```python
from build123d import *

# Parameters (mm, degrees)
F1_DEPTH = 6
F3_D     = 6
F4_W     = 63.5
F4_H     = 140
F5_DEPTH = 25


with BuildPart() as f1:
    # F0 (on Front) → F1 (new body)
    with BuildSketch(Plane.XZ):
        with BuildLine():
            Line((34.0407285993, 33.1888695754), (-82.9592714007, 33.1888695754))
            ThreePointArc((-82.9592714007, 33.1888695754), (-86.4948053066, 31.7244034814), (-87.9592714007, 28.1888695754))
            Line((-87.9592714007, 28.1888695754), (-87.9592714007, -99.5111304246))
            ThreePointArc((-87.9592714007, -99.5111304246), (-86.4948053066, -103.0466643305), (-82.9592714007, -104.5111304246))
            Line((-82.9592714007, -104.5111304246), (-57.5592714007, -104.5111304246))
            ThreePointArc((-57.5592714007, -104.5111304246), (-54.0237374948, -103.0466643305), (-52.5592714007, -99.5111304246))
            Line((-52.5592714007, -99.5111304246), (-52.5592714007, -91.8111304246))
            Line((-52.5592714007, -91.8111304246), (-62.5592714007, -91.8111304246))
            Line((-62.5592714007, -91.8111304246), (-62.5592714007, -16.8111304246))
            ThreePointArc((-62.5592714007, -16.8111304246), (-55.2369409303, 0.8665391051), (-37.5592714007, 8.1888695754))
            Line((-37.5592714007, 8.1888695754), (-11.3592714007, 8.1888695754))
            ThreePointArc((-11.3592714007, 8.1888695754), (6.318398129, 0.8665391051), (13.6407285993, -16.8111304246))
            Line((13.6407285993, -16.8111304246), (13.6407285993, -91.8111304246))
            Line((13.6407285993, -91.8111304246), (3.6407285993, -91.8111304246))
            Line((3.6407285993, -91.8111304246), (3.6407285993, -99.5111304246))
            ThreePointArc((3.6407285993, -99.5111304246), (5.1051946934, -103.0466643305), (8.6407285993, -104.5111304246))
            Line((8.6407285993, -104.5111304246), (34.0407285993, -104.5111304246))
            ThreePointArc((34.0407285993, -104.5111304246), (37.5762625052, -103.0466643305), (39.0407285993, -99.5111304246))
            Line((39.0407285993, -99.5111304246), (39.0407285993, 28.1888695754))
            ThreePointArc((39.0407285993, 28.1888695754), (37.5762625052, 31.7244034814), (34.0407285993, 33.1888695754))
        make_face()
    extrude(amount=F1_DEPTH)

    # F3 (through all)
    with Locations(Plane.XZ.offset(6)):
        with Locations((-75.2592714007, 20.6888695754), (-75.2592714007, -29.3111304246), (-75.2592714007, -79.3111304246), (-24.4592714007, 20.6888695754), (26.3407285993, 20.6888695754), (26.3407285993, -29.3111304246), (26.3407285993, -79.3111304246)):
            Hole(F3_D / 2)

    # F4 (on face) → F5 (cut)
    with BuildSketch(Plane.XZ.offset(6)):
        with Locations((7.2907285993, -36.8111304246)):
            Rectangle(F4_W, F4_H)
    extrude(amount=-F5_DEPTH, mode=Mode.SUBTRACT)


solid = f1.part
```
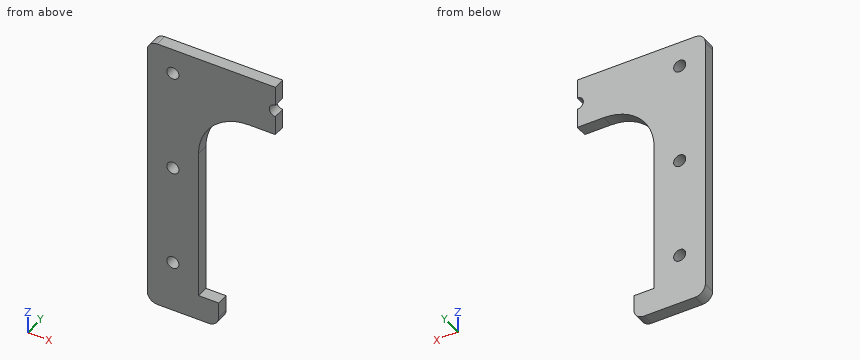
Check sheet for the modelled part. Datum: model origin and axes. Units: mm. Round coordinates to 2 decimals unless told otherwise and drop trailing zeros. Loops run counter-clockwise (first coordinate to the right, second up) from the corner with the lowest first, then second, coordinate; pieces in that order, holes last. Notation, with made-up numbers: (19.25, 89.25) - (46.25, 89.25) arc R29 ccw to (46.25, 114.25) - close; hole circle Ø2 at (21.25, 8.25). An arc over 180 degrees is marked (long way). Write item = value, one per line. Start each with the question number.
Q1. Depth check by flat-ended pin: P1, Ø7, axis at x = -75.26, z = -79.31, coming from the +Y side; P2, Ø2, axis at y = -4, z = -2, coming from the +X side; P3, Ø1, axis at y = -5, z = -67, coming from the +X side. Enter the tip coordinate at first touch or a pass-through.
Q2. Section check B-B (y = -3.05). Record the boundary of the cut face in (x, z), plus the area to 3 significant figures.
Q3. Section check C-C (x = -77). Record the boundary of the cut face in (y, z).
Q4. Section check A-A (x = -55.5). Record the boundary of the cut face in (y, z).
Q5. Section check D-D (z = -95). Record the boundary of the cut face in (x, y).
Q6. Thickness scan on L1, parallel to Z at x = -74, y = -0.95; L2, parallel to X at y = -0.85, z = 21; L3, parallel to X at y = -4.05, z = -86. Record the ranges inside material, lowest first.
Derived:
q1.P1 = 0
q1.P2 = -56.92
q1.P3 = -62.56
q2.outline = (-87.96, -99.51) arc R5 ccw to (-82.96, -104.51) - (-57.56, -104.51) arc R5 ccw to (-52.56, -99.51) - (-52.56, -91.81) - (-62.56, -91.81) - (-62.56, -16.81) arc R25 cw to (-37.56, 8.19) - (-24.46, 8.19) - (-24.46, 17.69) arc R3 cw to (-24.46, 23.69) - (-24.46, 33.19) - (-82.96, 33.19) arc R5 ccw to (-87.96, 28.19) - close; hole circle Ø6 at (-75.26, -79.31); hole circle Ø6 at (-75.26, -29.31); hole circle Ø6 at (-75.26, 20.69)
q2.area = 4,600 mm^2
q3.outline = (-6, -104.51) - (0, -104.51) - (0, -81.75) - (-6, -81.75) - close; (-6, -76.87) - (0, -76.87) - (0, -31.75) - (-6, -31.75) - close; (-6, -26.87) - (0, -26.87) - (0, 18.25) - (-6, 18.25) - close; (-6, 23.13) - (0, 23.13) - (0, 33.19) - (-6, 33.19) - close
q4.outline = (-6, -104.07) - (0, -104.07) - (0, -91.81) - (-6, -91.81) - close; (-6, 0.6) - (0, 0.6) - (0, 33.19) - (-6, 33.19) - close
q5.outline = (-87.96, -6) - (-52.56, -6) - (-52.56, 0) - (-87.96, 0) - close
q6.L1 = -104.51 to -82.03, -76.59 to -32.03, -26.59 to 17.97, 23.41 to 33.19
q6.L2 = -87.96 to -78.24, -72.28 to -27.44
q6.L3 = -87.96 to -62.56
